Geometry: final body of the model. Coordinates: model frame, mm. Coordinates: 2 decimals unless noted, no trailing zeros. Order: outer loops, then holes, each group sorted by start corner. A loop starts at its lowest first (then second) coordinate and runs counter-clockwise, first axis right, second up. Notation, with made-up numbers: (7.25, 67.25) -> (39.25, 67.25) arc R22 ccw to (39.25, 95.25) -> close; hole circle Ø6 at (-27, -17). An arc over 180 degrees is marked (long way). Answer in a Markdown table with one row per item. Add a question column.
1) Section query B-B on z = 0. Return the cut outline in (x, y), then the cut area to 3 significant figures.
2) Ray query, line 1 (X direction, y = 4.25, z = 0); line 2 (Z direction, x = 2.75, y = 8); line 3 (Z direction, x = 4.75, y = 120). Return the intervals inside material, ascending. Write a range as from..to.
3) Section query A-A on x = 0. Return the cut outline in (y, z), then the cut area to 3 significant figures.
4) Section query C-C on y = 52. Return the cut outline in (x, z), then the cut area to 3 significant figures.
5) Contact query for flat-ended pins moving along their axis: P1, Ø1, axis at x = -1.5, y = 131.5, coming from the -Z side; P2, Ø1.5, axis at x = 10, y = 37.5, coming from the +Z side; P3, Ø8, axis at x = 10.5, y = 48.5, coming from the +Z side. Output: stop coordinate, or through.
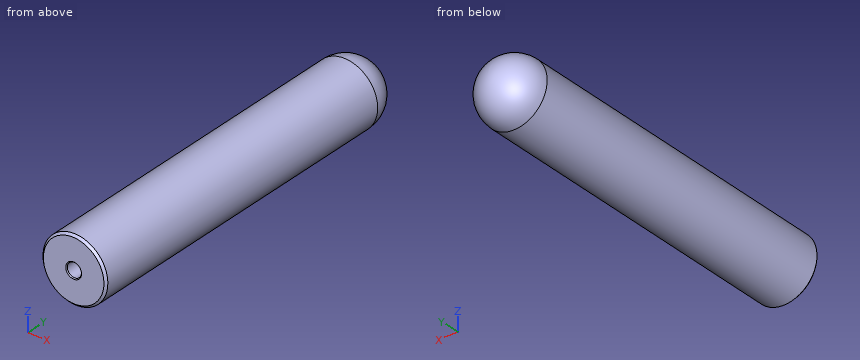
```python
from build123d import *

# Parameters (mm, degrees)
SKETCH1_R           = 15
BOSS_EXTRUDE1_DEPTH = 170
FILLET1_R           = 15
SKETCH2_R           = 3.25
CUT_EXTRUDE1_DEPTH  = 9.6
CHAMFER1_SIZE       = 0.4
CHAMFER2_SIZE       = 1


with BuildPart() as part:
    # Sketch1 → Boss-Extrude1 (new body)
    with BuildSketch(Plane(origin=(0, 0, 0), x_dir=(1, 0, 0), z_dir=(0, 1, 0))):
        with Locations(Location((0, 0, 0), (0, 0, 270))):
            Circle(SKETCH1_R)
    extrude(amount=BOSS_EXTRUDE1_DEPTH)

    # Fillet1
    fillet1_edges = [part.edges().sort_by_distance(p)[0] for p in [
        (0, 170, -15),
    ]]
    fillet(fillet1_edges, radius=FILLET1_R)

    # Sketch2 → Cut-Extrude1 (cut)
    with BuildSketch(Plane.XZ):
        with Locations(Location((0, 0, 0), (0, 0, 270))):
            Circle(SKETCH2_R)
    extrude(amount=-CUT_EXTRUDE1_DEPTH, mode=Mode.SUBTRACT)

    # Chamfer1
    chamfer1_edges = [part.edges().sort_by_distance(p)[0] for p in [
        (0, 0, 3.25),
    ]]
    chamfer(chamfer1_edges, length=CHAMFER1_SIZE)

    # Chamfer2
    chamfer2_edges = [part.edges().sort_by_distance(p)[0] for p in [
        (0, 0, -15),
    ]]
    chamfer(chamfer2_edges, length=CHAMFER2_SIZE)


solid = part.part
```
Result:
| question | item | result |
|---|---|---|
| 1 | outline | (-15, 1) -> (-14, 0) -> (-3.65, 0) -> (-3.25, 0.4) -> (-3.25, 9.6) -> (3.25, 9.6) -> (3.25, 0.4) -> (3.65, 0) -> (14, 0) -> (15, 1) -> (15, 155) arc R15 ccw to (-15, 155) -> close |
| 1 | area | 4,940 mm2 |
| 2 | line 1 | -15..-3.25, 3.25..15 |
| 2 | line 2 | -14.75..-1.73, 1.73..14.75 |
| 2 | line 3 | -14.23..14.23 |
| 3 | outline | (0, -14) -> (1, -15) -> (155, -15) arc R15 ccw to (155, 15) -> (1, 15) -> (0, 14) -> (0, 3.65) -> (0.4, 3.25) -> (9.6, 3.25) -> (9.6, -3.25) -> (0.4, -3.25) -> (0, -3.65) -> close |
| 3 | area | 4,940 mm2 |
| 4 | outline | circle Ø30 at (0, 0) |
| 4 | area | 707 mm2 |
| 5 | P1 | z = -14.97 |
| 5 | P2 | z = 11.81 |
| 5 | P3 | z = 13.52 |
